Build history of the part. All positions in model axes, mm. Face numbers are marked on the shaded views. A direction names the side the tool comes from. Round coordinates to 2 decimals unless told otherwise and drop trailing zeros. Write each loop counter-clockwise with the first axis right and the second up, starting at its lowest first coordinate (ties: lowest second). Pieces come first, ordered by that corner, then holes. Notation, with made-up numbers: M 28,-38.5 L 33,-38.5 A25 cw 33,-25.5 Z; hole C 65,-30.75 d2. An arc over 180 degrees is marked long. Use a Markdown table: item, result.
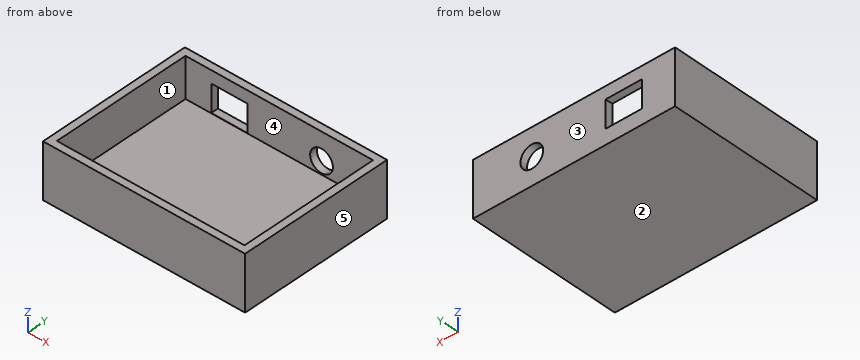
from build123d import *

# Parameters (mm, degrees)
F0_W     = 70.485
F0_H     = 53.975
F1_DEPTH = 19.05
F2_T     = -2.54
F3_W     = 12.7
F3_H     = 9.525
F4_DEPTH = 3.302
F6_D     = 7.9375
F6_DEPTH = 12.7
F6_TIP   = 2.3846655818
F7_DEPTH = 2.54


with BuildPart() as f1:
    # F0 (on Top) → F1 (new body)
    with BuildSketch(Plane.XY):
        Rectangle(F0_W, F0_H)
    extrude(amount=F1_DEPTH)

    # F2
    f2_openings = [f1.faces().sort_by_distance(p)[0] for p in [
        (0, 0, 19.05),
    ]]
    offset(amount=F2_T, openings=f2_openings)

    # F3 (on face) → F4 (cut)
    with BuildSketch(Plane(origin=(0, 26.9875, 0), x_dir=(-1, 0, 0), z_dir=(0, 1, 0))):
        with Locations((17.3686798662, 9.959281401)):
            Rectangle(F3_W, F3_H)
    extrude(amount=-F4_DEPTH, mode=Mode.SUBTRACT)

    # F6
    with Locations(Plane(origin=(0, 26.9875, 0), x_dir=(-1, 0, 0), z_dir=(0, 1, 0))):
        with Locations((-14.7299328819, 9.525)):
            Hole(F6_D / 2, depth=F6_DEPTH)
            with Locations((0, 0, -(F6_DEPTH + F6_TIP / 2))):  # 118° drill point
                Cone(0, F6_D / 2, F6_TIP, mode=Mode.SUBTRACT)

    # F7 (add): a face of the model
    f7_faces = [f1.faces().sort_by_distance(p)[0] for p in [
        (0, 0, 2.54),
    ]]
    extrude(f7_faces, amount=F7_DEPTH)


solid = f1.part
Q1. Cut at C-C on z = 8. Give the cut face in (x, y).
Response values:
| item | result |
|---|---|
| outline | M -35.24,-26.99 L 35.24,-26.99 L 35.24,26.99 L 18.39,26.99 L 18.39,24.45 L 32.7,24.45 L 32.7,-24.45 L -32.7,-24.45 L -32.7,24.45 L -23.72,24.45 L -23.72,26.99 L -35.24,26.99 Z; M -11.02,24.45 L 11.07,24.45 L 11.07,26.99 L -11.02,26.99 Z |
Q2. Drop flat-ended pins along their axis: P1, Ø10, axis at x = -25.5, y = -17, coming from the +Z side; P2, Ø7, axis at x = 14.73, z = 9.52, coming from the +Y side. Give the stop position or say it passes through.
Response values:
| item | result |
|---|---|
| P1 | stops at z = 5.08 |
| P2 | stops at y = -24.45 |
Q3. Which spindle directions (+Z, -Z, +X, -X, +Y, -Y) get a long thin tool onto all of the face, cutting with end or side? Do the marked faces 1 and 2. Say none if no direction does.
Response values:
| item | result |
|---|---|
| face 1 | +Z |
| face 2 | -Z, +X, -X, +Y, -Y |
Q4. Cut at A-A on x = -14. Give the cut face in (y, z).
Response values:
| item | result |
|---|---|
| outline | M -26.99,0 L 26.99,0 L 26.99,5.2 L 24.45,5.2 L 24.45,5.08 L -24.45,5.08 L -24.45,19.05 L -26.99,19.05 Z; M 24.45,14.72 L 26.99,14.72 L 26.99,19.05 L 24.45,19.05 Z |
Q5. Two-plate mould, pull along X, no slides. Class the marked faces 3, 4 and 5: +X half, -X half, draft (parallel to the pull), parting line (faces both ways), or undercut.
Response values:
| item | result |
|---|---|
| face 3 | draft |
| face 4 | undercut |
| face 5 | +X half |
Q6. Drill centre lines: L1, parallel to X at y = 17, z = 11.75; L2, parallel to Y at x = 22, z = 14.5; L3, parallel to Z at x = 8.5, y = -21. Where is each one in solid material? Low to high.
Response values:
| item | result |
|---|---|
| L1 | x = -35.24 to -32.7, 32.7 to 35.24 |
| L2 | y = -26.99 to -24.45, 24.45 to 26.99 |
| L3 | z = 0 to 5.08 |
Q7. Cut at B-B on z = 15.5. Give the cut face in (x, y), and give its area (3 significant figures).
Response values:
| item | result |
|---|---|
| outline | M -35.24,-26.99 L 35.24,-26.99 L 35.24,26.99 L -35.24,26.99 Z; hole M -32.7,-24.45 L 32.7,-24.45 L 32.7,24.45 L -32.7,24.45 Z |
| area | 606 mm2 |
Q8. Cut at D-D on y = 11. Give the cut face in (x, z).
Response values:
| item | result |
|---|---|
| outline | M -35.24,0 L 35.24,0 L 35.24,19.05 L 32.7,19.05 L 32.7,5.08 L -32.7,5.08 L -32.7,19.05 L -35.24,19.05 Z |
